Geometry check sheet. Reference: drawing and pictorial views, mm from the part's lowest x, y, z. A direction names the side the tool comes from. Round coordinates to 2 decimals unless told otherwise and drop trailing zeros. Write each loop counter-clockwise with the first axis right and the second up, starting at its lowest first coordinate (ties: lowest second). Pieces come first, ordered by that corner, then holes. Notation, with made-up numbers: (33, 15) -> (55, 15) arc R27 ccw to (55, 46) -> close; hole circle Ø1 at (21.25, 60.5). An arc over 180 degrees is marked (long way). Answer as a JSON object with one key per item and string values. Group by question number.
(1) Sectioned sample at A-A on y = 44.5. Record the cut outline in (x, z) (1 decimal).
(2) Scan lines: L1, parallel to X at y = 42, z = 52 (1 decimal); L2, parallel to Z at x = 28.5, y = 45 (1 decimal); L3, parallel to Z at x = 9, y = 48. Record each from-to range of solid material in increasing order. Write a range as from..to.
(3) Sectioned sample at C-C on x = 3. Record the cut outline in (y, z), and give its area (3 significant figures).
(4) Set-up check for the marked faces 5 and 6: record each of +Z, -Z, +X, -X, +Y, -Y from which the full face is reachable in a straight line by a thin tool's end or side.
(5) Sectioned sample at B-B on x = 37. Record the cut outline in (y, z).
(6) Gauge pin test, flat ends, axial feed: pin 1 Ø1.5 at (x, y) = (8.5, 33.5) entering from +Z (1 decimal); pin 2 Ø13 at (y, z) = (23.5, 24) entering from +X; pin 3 Ø4 at (x, y) = (18.5, 22) entering from -Z. Record the tip position at first contact, or that the pin passes through.
(7) Draft check along X on the marked faces 1, 2, 3 and 4. Enter one of: released by +X, released by -X, zero draft, split by the parting line, or undercut.
(8) Sectioned sample at D-D on z = 26.5. Record the cut outline in (x, y), and give its area (3 significant figures).
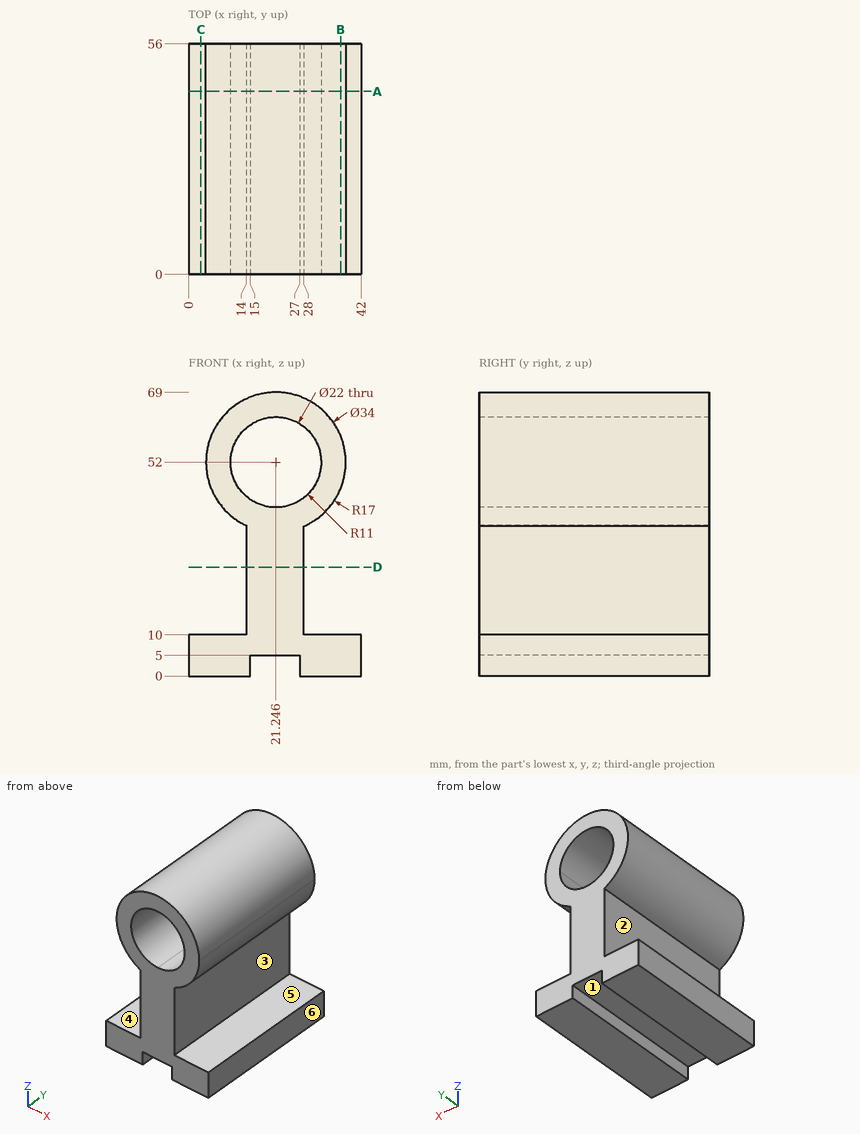
Computed values:
{
 "1": {"outline": "(0, 0) -> (15, 0) -> (15, 5) -> (27, 5) -> (27, 0) -> (42, 0) -> (42, 10) -> (28, 10) -> (28, 36.4) arc R17 ccw (long way) to (14, 36.6) -> (14, 10) -> (0, 10) -> close; hole (21.2, 41) arc R11 ccw to (32.2, 52) arc R11 ccw (long way) to start"},
 "2": {"L1": "4.2..10.2, 32.2..38.2", "L2": "0..10, 36.6..43.7, 60.3..67.4", "L3": "0..10, 40.21..63.79"},
 "3": {"outline": "(0, 0) -> (56, 0) -> (56, 10) -> (0, 10) -> close", "area": "560 mm2"},
 "4": {"face 5": "+X, +Y, -Y", "face 6": "+Z, -Z, +X, +Y, -Y"},
 "5": {"outline": "(0, 0) -> (56, 0) -> (56, 10) -> (0, 10) -> close; (0, 45.61) -> (56, 45.61) -> (56, 58.39) -> (0, 58.39) -> close"},
 "6": {"pin 1": "z = 64", "pin 2": "x = 28", "pin 3": "z = 5"},
 "7": {"face 1": "undercut", "face 2": "released by -X", "face 3": "released by +X", "face 4": "zero draft"},
 "8": {"outline": "(14, 0) -> (28, 0) -> (28, 56) -> (14, 56) -> close", "area": "784 mm2"}
}
